Part model, mm, in its own coordinate system. Give positions to 0.01 mm unless a question says otherwise; leave off trailing zeros. Order: outer loops, then holes, each group sorted by start corner. A loop starts at its lowest first (then second) coordinate and runs counter-clockwise, first axis right, second up. Notation, with made-up numbers: M 48.5,72.5 L 58.5,72.5 A28 cw 58.5,102.5 Z; hole C -18,51.5 d4. An arc over 180 degrees is marked long. Return JSON: item names as keys, results as strings.
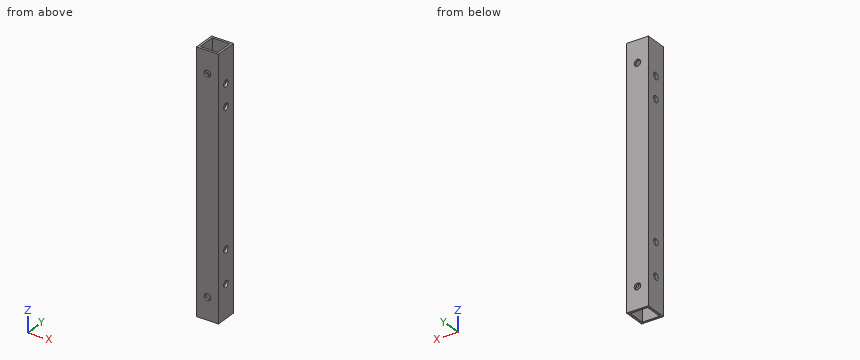
from build123d import *

# Parameters (mm, degrees)
SKETCH_1_W          = 10
SKETCH_1_H          = 10
SKETCH_1_W_2        = 8
SKETCH_1_H_2        = 8
EXTRUDE_1_DEPTH     = 117
SKETCH_2_R          = 1.5
CUT_EXTRUDE_1_DEPTH = 11
SKETCH_3_R          = 1.5
CUT_EXTRUDE_2_DEPTH = 10


with BuildPart() as part:
    # 草图1 → 拉伸-薄壁1 (new body)
    with BuildSketch(Plane.XY):
        Rectangle(SKETCH_1_W, SKETCH_1_H)
        Rectangle(SKETCH_1_W_2, SKETCH_1_H_2, mode=Mode.SUBTRACT)
    extrude(amount=EXTRUDE_1_DEPTH)

    # 草图2 → 切除-拉伸1 (cut, through all)
    with BuildSketch(Plane(origin=(0, 5, 0), x_dir=(1, 0, 0), z_dir=(0, 1, 0))):
        with Locations((0, -10)):
            Circle(SKETCH_2_R)
        with Locations((0, -107)):
            Circle(SKETCH_2_R)
    extrude(amount=-CUT_EXTRUDE_1_DEPTH, mode=Mode.SUBTRACT)

    # 草图3 → 切除-拉伸2 (cut)
    with BuildSketch(Plane(origin=(5, 0, 0), x_dir=(0, 0, -1), z_dir=(1, 0, 0))):
        with Locations((-15, 0)):
            Circle(SKETCH_3_R)
        with Locations((-30, 0)):
            Circle(SKETCH_3_R)
        with Locations((-102, 0)):
            Circle(SKETCH_3_R)
        with Locations((-92, 0)):
            Circle(SKETCH_3_R)
    extrude(amount=-CUT_EXTRUDE_2_DEPTH, mode=Mode.SUBTRACT)


solid = part.part
Q1. Band-saw the part on C-C (x = 0). Give the cut face in (y, z).
Established:
{"outline": "M -5,0 L -4,0 L -4,8.5 L -5,8.5 Z; M -5,11.5 L -4,11.5 L -4,105.5 L -5,105.5 Z; M -5,108.5 L -4,108.5 L -4,117 L -5,117 Z; M 4,0 L 5,0 L 5,8.5 L 4,8.5 Z; M 4,11.5 L 5,11.5 L 5,105.5 L 4,105.5 Z; M 4,108.5 L 5,108.5 L 5,117 L 4,117 Z"}
Q2. Band-saw the part on B-B (z = 30). Give the cut face in (x, y), then the cut area to 3 significant figures.
Established:
{"outline": "M -5,-5 L 5,-5 L 5,-1.5 L 4,-1.5 L 4,-4 L -4,-4 L -4,-1.5 L -5,-1.5 Z; M -5,1.5 L -4,1.5 L -4,4 L 4,4 L 4,1.5 L 5,1.5 L 5,5 L -5,5 Z", "area": "30.0 mm²"}
Q3. Band-saw the part on D-D (z = 91.5). Give the cut face in (x, y).
Established:
{"outline": "M -5,-5 L 5,-5 L 5,-1.41 L 4,-1.41 L 4,-4 L -4,-4 L -4,-1.41 L -5,-1.41 Z; M -5,1.41 L -4,1.41 L -4,4 L 4,4 L 4,1.41 L 5,1.41 L 5,5 L -5,5 Z"}
Q4. Band-saw the part on A-A (y = 2.5). Give the cut face in (x, z).
Established:
{"outline": "M -5,0 L -4,0 L -4,117 L -5,117 Z; M 4,0 L 5,0 L 5,117 L 4,117 Z"}
Q5. Probe line 1 along Z through (x, y) = (0, -4.4); line 2 along Y through (x, z) = (-4.55, 102); line 3 along Y through (x, z) = (1.5, 32). List the from-to ranges inside material, lowest first.
Established:
{"line 1": "z = 0 to 8.5, 11.5 to 105.5, 108.5 to 117", "line 2": "y = -5 to -1.5, 1.5 to 5", "line 3": "y = -5 to -4, 4 to 5"}
